from build123d import *

# Parameters (mm, degrees)
SKETCH1_R           = 1.25
BOSS_EXTRUDE1_DEPTH = 1


with BuildPart() as part:
    # Sketch1 → Boss-Extrude1 (new, symmetric)
    with BuildSketch(Plane(origin=(0, 0, 0), x_dir=(1, 0, 0), z_dir=(0, 1, 0))):
        with BuildLine():
            ThreePointArc((3, 5), (0, 8), (-3, 5))
            Line((-3, 5), (-2.973451327, 4.601769912))
            Line((-2.973451327, 4.601769912), (-2, -10))
            ThreePointArc((-2, -10), (0, -12), (2, -10))
            Line((2, -10), (2.973451327, 4.601769912))
            Line((2.973451327, 4.601769912), (3, 5))
        make_face()
        with Locations(Location((0, -10, 0), (0, 0, 270))):
            Circle(SKETCH1_R, mode=Mode.SUBTRACT)
        with Locations(Location((0, 5, 0), (0, 0, 270))):
            Circle(SKETCH1_R, mode=Mode.SUBTRACT)
    extrude(amount=BOSS_EXTRUDE1_DEPTH, both=True)


solid = part.part
Source: CAD feature listing. Evaluate the final solid. Frame: model axes, mm. Give positions to 0.01 mm unless a question says otherwise; leave off trailing zeros. Loops run counter-clockwise (first coordinate to the right, second up) from the corner with the lowest first, then second, coordinate; pieces in that order, holes last. Notation, with made-up numbers: (29.25, -15) -> (75.25, -15) arc R33 cw to (75.25, 18) -> close; hole circle Ø2 at (44, -11). An arc over 180 degrees is marked (long way). Use a Markdown table: item, result. Add a question column.
1) Line query: line 1 along X through (y, z) = (0.05, -5); line 2 along Z through (x, y) = (-0.25, 0.3); line 3 along X through (y, z) = (0.35, 10). Output: solid intervals per line, ascending. Write a range as [from, to].
2) Section query C-C, the plane y = -0.1. Return the cut outline in (x, z), then the cut area to 3 significant figures.
3) Section query D-D, the plane z = 8.5. Return the cut outline in (x, y), then the cut area to 3 significant figures.
4) Pull-direction query (X, two-part tool) for faces 1 (the face through (0, -1, 2)), 2 (the face through (0, 0, 12)), 3 (the face through (0.05, -0.01, -6.25)); classes: +X half, -X half, draft (parallel to the pull), parting line (faces both ways), or undercut.
5) Section query A-A, the plane x = 0. Return the cut outline in (y, z), then the cut area to 3 significant figures.
6) Section query B-B, the plane z = -5.5. Return the cut outline in (x, y), then the cut area to 3 significant figures.
Numbers:
| question | item | result |
|---|---|---|
| 1 | line 1 | x = [-3, -1.25], [1.25, 3] |
| 1 | line 2 | z = [-7.99, -6.22], [-3.78, 8.78], [11.22, 11.98] |
| 1 | line 3 | x = [-2, -1.25], [1.25, 2] |
| 2 | outline | (-3, -5) arc R3 ccw to (3, -5) -> (2, 10) arc R2 ccw to (-2, 10) -> close; hole circle Ø2.5 at (0, -5); hole circle Ø2.5 at (0, 10) |
| 2 | area | 85.6 mm2 |
| 3 | outline | (-2.1, -1) -> (2.1, -1) -> (2.1, 1) -> (-2.1, 1) -> close |
| 3 | area | 8.40 mm2 |
| 4 | face 1 | draft |
| 4 | face 2 | parting line |
| 4 | face 3 | undercut |
| 5 | outline | (-1, -8) -> (1, -8) -> (1, -6.25) -> (-1, -6.25) -> close; (-1, -3.75) -> (1, -3.75) -> (1, 8.75) -> (-1, 8.75) -> close; (-1, 11.25) -> (1, 11.25) -> (1, 12) -> (-1, 12) -> close |
| 5 | area | 30.0 mm2 |
| 6 | outline | (-2.96, -1) -> (-1.15, -1) -> (-1.15, 1) -> (-2.96, 1) -> close; (1.15, -1) -> (2.96, -1) -> (2.96, 1) -> (1.15, 1) -> close |
| 6 | area | 7.25 mm2 |
